```python
from build123d import *

# Parameters (mm, degrees)
F1_DEPTH = 31.75
F3_DEPTH = 12.7
F5_DEPTH = 12.7
F7_DEPTH = 12.7


with BuildPart() as f1:
    # F0 (on Top) → F1 (new body)
    with BuildSketch(Plane.XY):
        Polygon((0, 25.4), (0, 0), (12.7, 0), (12.7, 25.4), (25.4, 25.4), (25.4, 44.45), (-12.7, 44.45), (-12.7, 25.4), align=None)
    extrude(amount=-F1_DEPTH)

    # F2 (on face) → F3 (cut)
    with BuildSketch(Plane(origin=(-12.7, 0, 0), x_dir=(0, -1, 0), z_dir=(-1, 0, 0))):
        Polygon((-34.925, 0), (-25.4, -31.75), (-25.4, 0), align=None)
    extrude(amount=-F3_DEPTH, mode=Mode.SUBTRACT)

    # F4 (on face) → F5 (cut)
    with BuildSketch(Plane(origin=(0, 0, 0), x_dir=(0, -1, 0), z_dir=(-1, 0, 0))):
        Polygon((-13.476862, 0), (0, -31.75), (0, 0), align=None)
    extrude(amount=-F5_DEPTH, mode=Mode.SUBTRACT)

    # F6 (on face) → F7 (cut)
    with BuildSketch(Plane.YZ.offset(25.4)):
        Polygon((25.4, -31.75), (34.925, 0), (25.4, 0), align=None)
    extrude(amount=-F7_DEPTH, mode=Mode.SUBTRACT)


solid = f1.part
```
Here's how the part is built. I have some questions about the finished solid (model axes, mm). A direction names the side the tool comes from. Coordinates: 2 decimals unless noted, no trailing zeros. Order: outer loops, then holes, each group sorted by start corner. A loop starts at its lowest first (then second) coordinate and runs counter-clockwise, first axis right, second up. Notation, with made-up numbers: (70, 75.25) -> (95, 75.25) arc R21 cw to (95, 109.25) -> close; hole circle Ø4 at (-23.5, 71.5). An arc over 180 degrees is marked (long way). Return JSON: item names as keys, results as strings.
1) I'm going to push flat-ended pins straight in: P1, Ø9.5, axis at y = 16.5, z = -8.5, coming from the +X side; P2, Ø1.5, axis at x = 20, z = -28, coming from the -Y side. Where does each tip first touch, or does it pass through?
Conclusion:
{"P1": "stops at x = 12.7", "P2": "stops at y = 26.3"}
2) If we section it at D-D on y = 15: List the corners of the cut face in (x, z) for me.
Conclusion:
{"outline": "(0, -31.75) -> (12.7, -31.75) -> (12.7, 0) -> (0, 0) -> close"}
3) On a 3-axis mill with a long thin cutter (end or side, diameter ignored), from which of +Z, -Z, +X, -X, +Y, -Y can I reach the whole of each face in a straight line? I mean faces 1 (the flat face through (-12.7, 37, -16)), 2 (the flat face through (12.7, 17, -16)), 3 (the flat face through (0, 18, -16)). Say none if no direction works.
Conclusion:
{"face 1": "+Z, -Z, -X, +Y, -Y", "face 2": "+Z, +X, -Y", "face 3": "+Z, -X, -Y"}
4) Thinking about a two-plate mould opening in Y: for faces 4 (the flat face through (6, 27, -31.75)), 5 (the flat face through (6.261, 6.833, -15.653)), 6 (the flat face through (7, 44.45, -16)), which applies, +Y half, -Y half, draft (parallel to the pull), parting line (faces both ways), or undercut?
Conclusion:
{"face 4": "draft", "face 5": "-Y half", "face 6": "+Y half"}
5) If we section it at C-C on x = 8: List the corners of the cut face in (y, z) for me, plus the area to 3 significant figures.
Conclusion:
{"outline": "(0, -31.75) -> (44.45, -31.75) -> (44.45, 0) -> (13.48, 0) -> close", "area": "1,200 mm²"}
6) If I drill on probe 1 along X at (y, z) = (22.5, -19.5); probe 2 along Y at (x, z) = (11.5, -7); probe 3 along Y at (x, z) = (19, -9.5) (3 decimals), over which ranges is the centre line in solid material (lowest first)?
Conclusion:
{"probe 1": "x = 0 to 12.7", "probe 2": "y = 10.51 to 44.45", "probe 3": "y = 32.075 to 44.45"}
7) If we section it at B-B on z = -27.5: List the corners of the cut face in (x, y) for me (3 decimals), plus the area to 3 significant figures.
Conclusion:
{"outline": "(-12.7, 26.675) -> (0, 26.675) -> (0, 1.804) -> (12.7, 1.804) -> (12.7, 26.675) -> (25.4, 26.675) -> (25.4, 44.45) -> (-12.7, 44.45) -> close", "area": "993 mm²"}
8) If we section it at A-A on y = 33.5: List the corners of the cut face in (x, z) for me, plus the area to 3 significant figures.
Conclusion:
{"outline": "(-12.7, -31.75) -> (25.4, -31.75) -> (25.4, -4.75) -> (12.7, -4.75) -> (12.7, 0) -> (0, 0) -> (0, -4.75) -> (-12.7, -4.75) -> close", "area": "1,090 mm²"}
